Read the model definition and answer for the solid it produces. Units are mm, in the model's axes. Face numbers are marked on the shaded views. A direction names the side the tool comes from. Coordinates: 2 decimals unless noted, no trailing zeros. Order: outer loops, then holes, each group sorted by start corner. A loop starts at its lowest first (then second) coordinate and runs counter-clockwise, first axis right, second up. Notation, with made-up numbers: (47, 36.25) -> (51, 36.25) arc R18 ccw to (51, 54.25) -> close; hole circle Ø11 at (13, 17). An arc over 180 degrees is marked (long way). Answer in a Markdown table with one row per item.
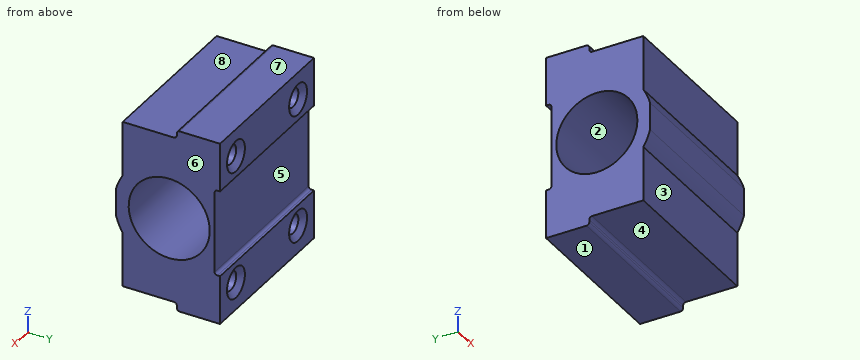
from build123d import *

# Parameters (mm, degrees)
SKETCH1_R                                         = 7.5
BOSS_EXTRUDE1_DEPTH                               = 30
CSK_FOR_4_FLAT_HEAD_MACHINE_SCREW_100_D           = 3.4544
CSK_FOR_4_FLAT_HEAD_MACHINE_SCREW_100_DEPTH       = 6.35
CSK_FOR_4_FLAT_HEAD_MACHINE_SCREW_100_CSINK_D     = 5.715
CSK_FOR_4_FLAT_HEAD_MACHINE_SCREW_100_CSINK_ANGLE = 100
CSK_FOR_4_FLAT_HEAD_MACHINE_SCREW_100_TIP         = 1.037806461
FILLET1_R                                         = 0.508


with BuildPart() as part:
    # Sketch1 → Boss-Extrude1 (new body)
    with BuildSketch(Plane(origin=(0, 0, 0), x_dir=(0, 0, -1), z_dir=(1, 0, 0))):
        with BuildLine():
            Line((32.5, 0), (34, 0))
            Line((34, 0), (34, 7.49375))
            Line((34, 7.49375), (34, 8))
            Line((34, 8), (25, 8))
            Line((25, 8), (25, 7))
            Line((25, 7), (9, 7))
            Line((9, 7), (9, 8))
            Line((9, 8), (0, 8))
            Line((0, 8), (0, 7.49375))
            Line((0, 7.49375), (0, 0))
            Line((0, 0), (1.5, 0))
            Line((1.5, 0), (1.5, -10))
            Line((1.5, -10), (11.611411797, -10))
            ThreePointArc((11.611411797, -10), (13.001010498, -10.730169916), (14.486500092, -11.237568497))
            Line((14.486500092, -11.237568497), (19.549499908, -11.237568497))
            ThreePointArc((19.549499908, -11.237568497), (21.034989502, -10.730169916), (22.424588203, -10))
            Line((22.424588203, -10), (32.5, -10))
            Line((32.5, -10), (32.5, 0))
        make_face()
        with Locations((17.018, -1.398)):
            Circle(SKETCH1_R, mode=Mode.SUBTRACT)
    extrude(amount=BOSS_EXTRUDE1_DEPTH)

    # CSK for #4 Flat Head Machine Screw (100)1
    with Locations(Plane(origin=(0, 8, 0), x_dir=(1, 0, 0), z_dir=(0, 1, 0))):
        with Locations((5.08, 28.92), (24.92, 28.92), (24.92, 5.08), (5.08, 5.08)):
            CounterSinkHole(CSK_FOR_4_FLAT_HEAD_MACHINE_SCREW_100_D / 2, CSK_FOR_4_FLAT_HEAD_MACHINE_SCREW_100_CSINK_D / 2, depth=CSK_FOR_4_FLAT_HEAD_MACHINE_SCREW_100_DEPTH, counter_sink_angle=CSK_FOR_4_FLAT_HEAD_MACHINE_SCREW_100_CSINK_ANGLE)
            with Locations((0, 0, -(CSK_FOR_4_FLAT_HEAD_MACHINE_SCREW_100_DEPTH + CSK_FOR_4_FLAT_HEAD_MACHINE_SCREW_100_TIP / 2))):  # 118° drill point
                Cone(0, CSK_FOR_4_FLAT_HEAD_MACHINE_SCREW_100_D / 2, CSK_FOR_4_FLAT_HEAD_MACHINE_SCREW_100_TIP, mode=Mode.SUBTRACT)

    # Fillet1
    fillet1_edges = [part.edges().sort_by_distance(p)[0] for p in [
        (15, 7, -9),
        (15, 7, -25),
        (15, 0, -34),
        (15, 0, -32.5),
        (15, 0, -1.5),
        (15, 0, 0),
    ]]
    fillet(fillet1_edges, radius=FILLET1_R)


solid = part.part
Q1. Consider line 1 (X direction, y = 4.65, z = -28.92); line 2 (Z direction, x = 24.92, y = 4.2); line 3 (Z direction, x = 5.08, y = 4.8). Determine where each line is inside the solid, lowest interval first.
Outcome:
| item | result |
|---|---|
| line 1 | 0 to 3.35, 6.81 to 23.19, 26.65 to 30 |
| line 2 | -34 to -30.65, -27.19 to -22.01, -12.03 to -6.81, -3.35 to 0 |
| line 3 | -34 to -30.65, -27.19 to -21.24, -12.79 to -6.81, -3.35 to 0 |
Q2. Given pin 1 (2 mm diameter, centred on x = 24.5, z = -15.5, fed in from +Y); pin 2 (1.5 mm diameter, centred on x = 26, z = -24.5, fed in from -Y); pin 3 (0.5 mm diameter, centred on x = 18.5, z = -33, fed in from -Y); pin 4 (8 mm diameter, centred on x = 21, z = -24, fed in from +Y), each flat-ended and moving along its own axis, determine where each tip first touches the part or whether it passes through.
Outcome:
| item | result |
|---|---|
| pin 1 | y = 7 |
| pin 2 | y = -10 |
| pin 3 | y = -0.07 |
| pin 4 | y = 8 |
Q3. For the marked faces 4, 5, 6, 7 and 8, determine the directions among +Z, -Z, +X, -X, +Y, -Y from which every point of the face is accessible in a straight line to the end or side of a thin tool.
Outcome:
| item | result |
|---|---|
| face 4 | -Z, +X, -X, -Y |
| face 5 | +X, -X, +Y |
| face 6 | +Z, -Z, +X, +Y, -Y |
| face 7 | +Z, +X, -X, +Y, -Y |
| face 8 | +Z, +X, -X, -Y |
Q4. The part is cut by section C-C (z = -15.5). Write down the section's boundary in (x, y).
Outcome:
| item | result |
|---|---|
| outline | (0, -11.24) -> (30, -11.24) -> (30, -8.74) -> (0, -8.74) -> close; (0, 5.95) -> (30, 5.95) -> (30, 7) -> (0, 7) -> close |
Q5. The part is cut by section B-B (x = 12.75). Write down the section's boundary in (y, z).
Outcome:
| item | result |
|---|---|
| outline | (-11.24, -19.55) arc R10.16 ccw to (-10, -22.42) -> (-10, -32.5) -> (-0.51, -32.5) arc R0.51 cw to (0, -33.01) -> (0, -33.49) arc R0.51 ccw to (0.51, -34) -> (8, -34) -> (8, -25) -> (7.51, -25) arc R0.51 cw to (7, -24.49) -> (7, -9.51) arc R0.51 cw to (7.51, -9) -> (8, -9) -> (8, 0) -> (0.51, 0) arc R0.51 ccw to (0, -0.51) -> (0, -0.99) arc R0.51 cw to (-0.51, -1.5) -> (-10, -1.5) -> (-10, -11.61) arc R10.16 ccw to (-11.24, -14.49) -> close; hole circle Ø15 at (-1.4, -17.02) |
Q6. For a pull along Y with two mould halves and no side action, classify the marked faces 1, 2 and 3 as pulls with the +Y half, pulls with the -Y half, needs draft (parallel to the pull), parting line crosses it, or undercut.
Outcome:
| item | result |
|---|---|
| face 1 | needs draft |
| face 2 | undercut |
| face 3 | pulls with the -Y half |
Q7. The part is cut by section A-A (z = -20). Write down the section's boundary in (x, y).
Outcome:
| item | result |
|---|---|
| outline | (0, -11.11) -> (30, -11.11) -> (30, -8.28) -> (0, -8.28) -> close; (0, 5.48) -> (30, 5.48) -> (30, 7) -> (0, 7) -> close |
